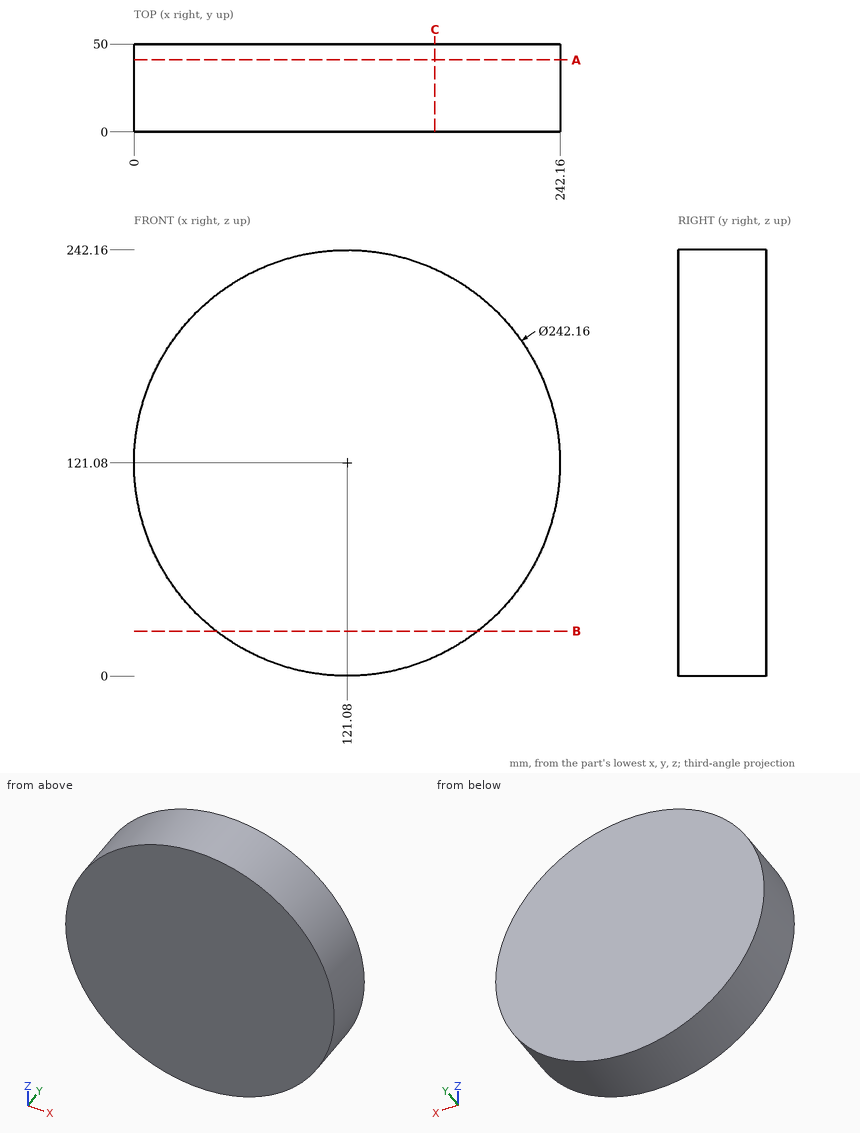
Print and shaded views of the part. All mm, measured from the part's lowest x, y and z. Round coordinates to 2 decimals unless told otherwise and drop trailing zeros. Write each loop counter-clockwise with the first axis right and the second up, starting at its lowest first coordinate (ties: lowest second). Pieces come first, ordered by that corner, then holes.
Item 1: Cut at A-A, the plane y = 41. Give the cut face in (x, z).
Results:
outline: circle Ø242.16 at (121.08, 121.08)
Item 2: Probe L1, parallel to Z at x = 57, y = 28; L2, parallel to X at y = 45.5, z = 139; L3, parallel to X at y = 28, z = 161.5. List the from-to ranges inside material, lowest first.
Results:
L1: z = 18.35 to 223.81
L2: x = 1.33 to 240.83
L3: x = 6.95 to 235.21
Item 3: Drop flat-ended pins along their axis: pin 1 Ø12 at (x, y) = (159.5, 21.5) entering from -Z; pin 2 Ø3 at (x, y) = (104.5, 9) entering from +Z; pin 3 Ø10 at (x, y) = (82, 30) entering from +Z; pin 4 Ø3 at (x, z) = (213.5, 111) entering from -Y. Give the stop position or say it passes through.
Results:
pin 1: stops at z = 4.42
pin 2: stops at z = 241.22
pin 3: stops at z = 237.26
pin 4: stops at y = 0
Item 4: Cut at C-C, the plane x = 171. Give the cut face in (y, z), plus the area to 3 significant figures.
Results:
outline: (0, 10.77) - (50, 10.77) - (50, 231.39) - (0, 231.39) - close
area: 11,000 mm2
Item 5: Cut at B-B, the plane z = 25.5. Give the cut face in (x, y).
Results:
outline: (46.75, 0) - (195.41, 0) - (195.41, 50) - (46.75, 50) - close
